```python
from build123d import *

# Parameters (mm, degrees)
F0_R      = 85
F3_R      = 142.5
F3_R_2    = 11
F3_R_3    = 85
F4_DEPTH  = 25
F5_R      = 110
F8_SIZE   = 21
F9_R      = 170
F9_R_2    = 11
F9_R_3    = 110
F10_DEPTH = 12.5


with BuildPart() as f2:
    # F2: sweep along a path in F1
    with BuildLine(Plane.XZ) as f2_path:
        Line((0, 0), (0, 70))
        ThreePointArc((0, 70), (-52.7207793864, 197.2792206136), (-180, 250))
        Line((-180, 250), (-1000, 250))
    # F0 (on Top) → F2 (sweep)
    with BuildSketch(Plane.XY):
        Circle(F0_R)
    sweep(path=f2_path.line)

    # F3 (on face) → F4 (join)
    with BuildSketch(Plane(origin=(0, 0, 0), x_dir=(1, 0, 0), z_dir=(0, 0, -1))):
        Circle(F3_R)
        with Locations((-84.8528137424, -84.8528137424)):
            Circle(F3_R_2, mode=Mode.SUBTRACT)
        with Locations((0, -120)):
            Circle(F3_R_2, mode=Mode.SUBTRACT)
        with Locations((84.8528137424, -84.8528137424)):
            Circle(F3_R_2, mode=Mode.SUBTRACT)
        with Locations((-120, 0)):
            Circle(F3_R_2, mode=Mode.SUBTRACT)
        with Locations((-84.8528137424, 84.8528137424)):
            Circle(F3_R_2, mode=Mode.SUBTRACT)
        Circle(F3_R_3, mode=Mode.SUBTRACT)
        with Locations((120, 0)):
            Circle(F3_R_2, mode=Mode.SUBTRACT)
        with Locations((0, 120)):
            Circle(F3_R_2, mode=Mode.SUBTRACT)
        with Locations((84.8528137424, 84.8528137424)):
            Circle(F3_R_2, mode=Mode.SUBTRACT)
    extrude(amount=-F4_DEPTH)

    # F7: sweep along a path in F6
    with BuildLine(Plane.XZ) as f7_path:
        Line((-2018.191576004, 0), (-2018.191576004, 50))
        ThreePointArc((-2018.191576004, 50), (-1959.6129322413, 191.4213562373), (-1818.191576004, 250))
        Line((-1818.191576004, 250), (-964.0375375748, 250))
    # F5 (on Top) → F7 (sweep)
    with BuildSketch(Plane.XY):
        with Locations((-2014.44, 0)):
            Circle(F5_R)
    sweep(path=f7_path.line)

    # F8
    f8_edges = [f2.edges().sort_by_distance(p)[0] for p in [
        (-964.037538, 0, 356.248424),
    ]]
    chamfer(f8_edges, length=F8_SIZE)

    # F9 (on face) → F10 (join, symmetric)
    with BuildSketch(Plane(origin=(0, 0, 0), x_dir=(1, 0, 0), z_dir=(0, 0, -1))):
        with Locations((-2014.44, 0)):
            Circle(F9_R)
        with Locations((-2118.738250225, -104.298250225)):
            Circle(F9_R_2, mode=Mode.SUBTRACT)
        with Locations((-2014.44, -147.5)):
            Circle(F9_R_2, mode=Mode.SUBTRACT)
        with Locations((-1910.141749775, -104.298250225)):
            Circle(F9_R_2, mode=Mode.SUBTRACT)
        with Locations((-2161.94, 0)):
            Circle(F9_R_2, mode=Mode.SUBTRACT)
        with Locations((-2118.738250225, 104.298250225)):
            Circle(F9_R_2, mode=Mode.SUBTRACT)
        with Locations((-2014.44, 0)):
            Circle(F9_R_3, mode=Mode.SUBTRACT)
        with Locations((-1866.94, 0)):
            Circle(F9_R_2, mode=Mode.SUBTRACT)
        with Locations((-2014.44, 147.5)):
            Circle(F9_R_2, mode=Mode.SUBTRACT)
        with Locations((-1910.141749775, 104.298250225)):
            Circle(F9_R_2, mode=Mode.SUBTRACT)
    extrude(amount=F10_DEPTH, both=True)


solid = f2.part
```
Input: part model. Units: mm. Frame: model coordinates. A direction names the side the tool comes from. Give positions to 0.01 mm unless a question says otherwise; leave off trailing zeros. Order: outer loops, then holes, each group sorted by start corner. A loop starts at its lowest first (then second) coordinate and runs counter-clockwise, first axis right, second up. Notation, with made-up numbers: M -15.75,72 L 24.25,72 A27 ccw 24.25,97 Z; hole C -3,43.25 d8. An arc over 180 degrees is marked long. One line per question, with ' | ' between items.
1) Access query for faces 1 (the face through (-1903, -2, -12.5)), 2 (the face through (-577.507, 25.532, 331.075)), 3 (the face through (-2184.276, -7.475, -0.175)). Directions: +Z, -Z, +X, -X, +Y, -Y. A direction counts if a zero-diameter tool reaches every point of the face in a straight line with its end or side. Return the directions, or none.
Filled in:
face 1: -Z, +X, -X, +Y, -Y | face 2: none | face 3: -Z
2) Draft query along Y for faces 4 (the face through (-1912.828, -42.131, 31.512)), 5 (the face through (-2, -2, 0)), 6 (the face through (-2016, 2, 0)). Return one class per face: pulls with the +Y half, pulls with the -Y half, needs draft (parallel to the pull), parting line crosses it, or undercut.
Filled in:
face 4: parting line crosses it | face 5: needs draft | face 6: undercut
3) Section A-A on x = -1051. Output: boundary loops of the cut face in (y, z), and give its area (3 significant figures).
Filled in:
outline: C 0,246.25 d220 | area: 38,000 mm2
4) Ray query, L1, parallel to Y at x = -2014.44, z = -3.5; L2, parallel to X at y = 0, z = 0.5; L3, parallel to X at y = 0, z = -5.25. Return the intervals inside material, ascending.
Filled in:
L1: y = -170 to -158.5, -136.5 to -110, 110 to 136.5, 158.5 to 170 | L2: x = -2184.44 to -2172.94, -2150.94 to -1877.94, -1855.94 to -1844.44, -142.5 to -131, -109 to 109, 131 to 142.5 | L3: x = -2184.44 to -2172.94, -2150.94 to -2124.44, -1904.44 to -1877.94, -1855.94 to -1844.44
5) Contact query for flat-ended pins moving along their axis: P1, Ø10, axis at x = -1612.5, y = 39, coming from the -Z side; P2, Ø5, axis at x = -1869, z = 275.5, coming from the -Y side; P3, Ø4, axis at y = 15, z = 61, coming from the +X side. Output: stop coordinate, or through.
Filled in:
P1: stops at z = 141.63 | P2: stops at y = -105.12 | P3: stops at x = 84
